The model under review builds one solid part; all positions refer to its coordinate system, in mm. A direction names the side the tool comes from. Coordinates: 2 decimals unless noted, no trailing zeros. Order: outer loops, then holes, each group sorted by start corner. A loop starts at its lowest first (then second) coordinate and runs counter-clockwise, first axis right, second up. Notation, with made-up numbers: M -20.75,27.5 L 29.25,27.5 A14 ccw 29.25,33.5 Z; hole C -12,-16.5 d10. An arc over 180 degrees is marked long. One line per item, written item: value.
```python
from build123d import *

# Parameters (mm, degrees)
SKETCH1_R                                           = 16
BOSS_EXTRUDE1_DEPTH                                 = 4
CUT_EXTRUDE2_DEPTH                                  = 2
SKETCH3_R                                           = 4.1
CUT_EXTRUDE1_DEPTH                                  = 23.978250586
CSK_FOR_M3_COUNTERSUNK_FLAT_HEAD_SCREW1_D           = 3.4
CSK_FOR_M3_COUNTERSUNK_FLAT_HEAD_SCREW1_CSINK_D     = 6.3
CSK_FOR_M3_COUNTERSUNK_FLAT_HEAD_SCREW1_CSINK_ANGLE = 90
BOSS_EXTRUDE3_DEPTH                                 = 4
FILLET3_R                                           = 20
BOSS_EXTRUDE4_DEPTH                                 = 10
CHAMFER1_SIZE                                       = 5
CUT_EXTRUDE5_DEPTH                                  = 74.993512369
SKETCH10_R                                          = 1.6
CUT_EXTRUDE4_DEPTH                                  = 77.518232271


with BuildPart() as part:
    # Sketch1 → Boss-Extrude1 (new body)
    with BuildSketch(Plane(origin=(0, 0, 0), x_dir=(0, 0, -1), z_dir=(1, 0, 0))):
        Circle(SKETCH1_R)
    extrude(amount=BOSS_EXTRUDE1_DEPTH)

    # Sketch5 → Cut-Extrude2 (cut)
    with BuildSketch(Plane(origin=(4, 0, 0), x_dir=(0, 0, -1), z_dir=(1, 0, 0))):
        with BuildLine():
            Line((-1.889696865, 12.6976), (-2.933047351, 2.719785513))
            ThreePointArc((-2.933047351, 2.719785513), (-4, 0), (-2.933047351, -2.719785513))
            Line((-2.933047351, -2.719785513), (-1.889696865, -12.6976))
            ThreePointArc((-1.889696865, -12.6976), (0, -14.4), (1.889696865, -12.6976))
            Line((1.889696865, -12.6976), (2.933047351, -2.719785513))
            ThreePointArc((2.933047351, -2.719785513), (4, 0), (2.933047351, 2.719785513))
            Line((2.933047351, 2.719785513), (1.889696865, 12.6976))
            ThreePointArc((1.889696865, 12.6976), (0, 14.4), (-1.889696865, 12.6976))
        make_face()
    extrude(amount=-CUT_EXTRUDE2_DEPTH, mode=Mode.SUBTRACT)

    # Sketch3 → Cut-Extrude1 (cut, through all)
    with BuildSketch(Plane(origin=(4, 0, 0), x_dir=(0, 0, -1), z_dir=(1, 0, 0))):
        Circle(SKETCH3_R)
    extrude(amount=-CUT_EXTRUDE1_DEPTH, mode=Mode.SUBTRACT)

    # CSK for M3 Countersunk Flat Head Screw1 (through all)
    with Locations(Plane.ZY):
        with Locations((-10, 0), (10, 0)):
            CounterSinkHole(CSK_FOR_M3_COUNTERSUNK_FLAT_HEAD_SCREW1_D / 2, CSK_FOR_M3_COUNTERSUNK_FLAT_HEAD_SCREW1_CSINK_D / 2, counter_sink_angle=CSK_FOR_M3_COUNTERSUNK_FLAT_HEAD_SCREW1_CSINK_ANGLE)

    # Sketch9 → Boss-Extrude3 (add)
    with BuildSketch(Plane(origin=(0, 0, 0), x_dir=(0, 0, -1), z_dir=(1, 0, 0))):
        with BuildLine():
            Line((-30.381570905, -7.754153907), (-30.381570905, -66))
            Line((-30.381570905, -66), (-15.381570905, -66))
            Line((-15.381570905, -66), (-15.381570905, -16))
            Line((-15.381570905, -16), (0, -16))
            ThreePointArc((0, -16), (-14.78207252, -6.122934918), (-11.313708499, 11.313708499))
            Line((-11.313708499, 11.313708499), (-30.381570905, -7.754153907))
        make_face()
    extrude(amount=BOSS_EXTRUDE3_DEPTH)

    # Fillet3
    fillet3_edges = [part.edges().sort_by_distance(p)[0] for p in [
        (2, -7.754153907, 30.381570905),
        (2, -16, 15.381570905),
    ]]
    fillet(fillet3_edges, radius=FILLET3_R)

    # Sketch11 → Boss-Extrude4 (add)
    with BuildSketch(Plane.XZ.offset(66)):
        Polygon((0, 15.381570905), (-10, 15.381570905), (-10, 0), (-20, 0), (-20, 30.381570905), (0, 30.381570905), align=None)
    extrude(amount=-BOSS_EXTRUDE4_DEPTH)

    # Chamfer1
    chamfer1_edges = [part.edges().sort_by_distance(p)[0] for p in [
        (-10, -61, 15.381570905),
        (-20, -61, 30.381570905),
        (0, -56, 22.881570905),
    ]]
    chamfer(chamfer1_edges, length=CHAMFER1_SIZE - 0.0001)  # a hair under: the kernel refuses the full size

    # Sketch12 → Cut-Extrude5 (cut, through all)
    with BuildSketch(Plane(origin=(-10, 0, 0), x_dir=(0, 0, -1), z_dir=(1, 0, 0))):
        Polygon((-6.955897301, -66), (-3.316194958, -56), (0, -56), (0, -66), align=None)
    extrude(amount=-CUT_EXTRUDE5_DEPTH, mode=Mode.SUBTRACT)

    # Sketch10 → Cut-Extrude4 (cut, through all)
    with BuildSketch(Plane(origin=(4, 0, 0), x_dir=(0, 0, -1), z_dir=(1, 0, 0))):
        with Locations((-22.881570905, -16)):
            Circle(SKETCH10_R)
        with Locations((-22.881570905, -31)):
            Circle(SKETCH10_R)
        with Locations((-22.881570905, -46)):
            Circle(SKETCH10_R)
        with Locations((-22.881570905, -61)):
            Circle(SKETCH10_R)
    extrude(amount=-CUT_EXTRUDE4_DEPTH, mode=Mode.SUBTRACT)


solid = part.part
```
(1) Tool access review of faces 1 (the flat face through (4, -15, 13)), 2 (the flat face through (-12, -56, 17)), 3 (the flat face through (3.01, -7.72, 2.41)): name each direction out of +Z, -Z, +X, -X, +Y, -Y from which nothing blocks a thin tool from reaching the whole face with its end or side.
Geometry results:
face 1: +Z, -Z, +X, +Y, -Y
face 2: +Z, -Z, -X, +Y
face 3: +X
(2) We need section A-A, the plane z = -10. State the section outline as (x, y) points.
Geometry results:
outline: M 0,-12.49 L 4,-12.49 L 4,-1.7 L 1.45,-1.7 L 0,-3.15 Z; M 0,3.15 L 1.45,1.7 L 4,1.7 L 4,12.49 L 0,12.49 Z
(3) We need section D-D, the plane x = -8.5. State the section outline as (y, z) points.
Geometry results:
outline: M -66,11.88 L -56,11.88 L -56,30.38 L -66,30.38 Z; hole C -61,22.88 d3.2
(4) We need section B-B, the plane y = -46. State the section outline as (x, z) points.
Geometry results:
outline: M 0,15.38 L 4,15.38 L 4,21.28 L 0,21.28 Z; M 0,24.48 L 4,24.48 L 4,30.38 L 0,30.38 Z
(5) We need section C-C, the plane y = 0. State the section outline as (x, z) points.
Geometry results:
outline: M 0,-16 L 4,-16 L 4,-11.7 L 1.45,-11.7 L 0,-13.15 Z; M 0,-6.85 L 1.45,-8.3 L 4,-8.3 L 4,-4.1 L 0,-4.1 Z; M 0,4.1 L 4,4.1 L 4,8.3 L 1.45,8.3 L 0,6.85 Z; M 0,13.15 L 1.45,11.7 L 4,11.7 L 4,22.63 L 0,22.63 Z
(6) For L1, parallel to Z at x = 2.75, y = -55; L2, parallel to Y at x = -14, z = 10.5; L3, parallel to Y at x = 2.3, z = 10, list the stretches that pass through material, from the lowest coordinate up.
Geometry results:
L1: z = 15.38 to 30.38
L2: y = -66 to -56
L3: y = -22.05 to -1.7, 1.7 to 12.49
(7) Insertion check: pin 1 Ø5.5 at (y, z) = (-60.5, 6.5) entering from +X; pin 2 Ø10 at (x, y) = (-0.5, -46.5) entering from -Z; pin 3 Ø12 at (x, z) = (-3, -10) entering from -Y; pin 4 Ø4 at (y, z) = (-31, 22.88) entering from +X. Each pin has a flat end and moves straight along its axis. Give the tip position at first contact, or say it passes through.
Geometry results:
pin 1: stops at x = -10
pin 2: stops at z = 15.38
pin 3: stops at y = -15.26
pin 4: stops at x = 4
(8) Mouldability with a two-part tool opening along Y and no side actions: class faces 4 (the cylindrical face through (1.584, 0.18, 4.096)), 5 (the flat face through (1.97, 4.8, 17.83)), 6 (the flat face through (3.014, 7.859, 2.396)), 7 (the flat face through (1, -52, 30.382)) as +Y half, -Y half, draft (parallel to the pull), parting line (faces both ways), or undercut.
Geometry results:
face 4: undercut
face 5: +Y half
face 6: undercut
face 7: draft
